Could you check a few things on this model? Use its own coordinates, in mm. A direction names the side the tool comes from. Round coordinates to 2 decimals unless told otherwise and drop trailing zeros. Write each loop counter-clockwise with the first axis right and the second up, starting at its lowest first coordinate (ties: lowest second). Pieces come first, ordered by that corner, then holes. Notation, with made-up numbers: M 5.5,-34 L 41.5,-34 A26 cw 41.5,-12 Z; hole C 82,-19.75 d4. An arc over 180 degrees is marked long. One line per item, written item: value. Start each with the question number.
(1) Thinking about a two-plate mould opening in X: for faces 6 (the face through (-42.005, 1, 0)), 7 (the face through (24.096, 1.493, 21.203)), 8 (the face through (3, 2, -20)), 9 (the face through (41.254, 0.986, 22.962)), which applies, released by +X, released by -X, zero draft, split by the parting line, or undercut?
(2) I'm going to push flat-ended pins straight in: pin 1 Ø0.9 at (x, z) = (-25.5, -20.5) entering from -Y; pin 2 Ø0.8 at (x, y) = (-35.5, 1.5) entering from +Z. Where does each tip first touch, or does it pass through?
(3) I want a section at B-B on z = -6. Please give me the cut outline in (x, y), and give its area (3 significant figures).
(4) If I drill on L1, parallel to X at y = 0.4, z = -9; L2, parallel to Z at x = 12, y = 1.4; L3, parallel to X at y = 1.15, z = 19, over which ranges is the centre line in solid material (lowest first)?
(5) Which directions (+Z, -Z, +X, -X, +Y, -Y) give clear straight access to the entire face, cutting with the end or side of a thin tool? Please do faces 1 (the face through (7, 1, 23.743)), 2 (the face through (-38.63, 1.493, 15.816)), 3 (the face through (1, 1, -22)), 4 (the face through (-41.224, 0.986, 23.002)), 5 (the face through (33.093, 0.986, -17.402)).
(6) I want a section at C-C on y = 0.6. Please give me the cut outline in (x, z).
(7) I want a section at A-A on x = -4.5. Please give me the cut outline in (y, z), and give its area (3 significant figures).
```python
from build123d import *

# Parameters (mm, degrees)
SKETCH_1_R          = 0.9
EXTRUDE_1_DEPTH     = 2
SKETCH_8_W          = 12
SKETCH_8_H          = 10.026739303
CUT_EXTRUDE_4_DEPTH = 1
SKETCH_9_R          = 1.5
CUT_EXTRUDE_7_DEPTH = 1
FILLET_1_R          = 2
SKETCH_10_W         = 12
SKETCH_10_H         = 6.28269209
CUT_EXTRUDE_8_DEPTH = 2
FILLET_2_R          = 1


with BuildPart() as part:
    # 草图1 → 凸台-拉伸1 (new body)
    with BuildSketch(Plane(origin=(0, 0, 0), x_dir=(1, 0, 0), z_dir=(0, 1, 0))):
        with BuildLine():
            Line((-39.407613887, 24.257383456), (39.397836405, 24.257383456))
            ThreePointArc((39.397836405, 24.257383456), (41.234387067, 23.496659264), (41.995111259, 21.660108602))
            Line((41.995111259, 21.660108602), (41.995111259, -21.14534169))
            ThreePointArc((41.995111259, -21.14534169), (41.234387067, -22.981892352), (39.397836405, -23.742616544))
            Line((39.397836405, -23.742616544), (-39.407613887, -23.742616544))
            ThreePointArc((-39.407613887, -23.742616544), (-41.244164549, -22.981892352), (-42.004888741, -21.14534169))
            Line((-42.004888741, -21.14534169), (-42.004888741, 21.660108602))
            ThreePointArc((-42.004888741, 21.660108602), (-41.244164549, 23.496659264), (-39.407613887, 24.257383456))
        make_face()
        with Locations((-25.004888281, 21.257382356)):
            Circle(SKETCH_1_R, mode=Mode.SUBTRACT)
        with Locations((-0.004887481, 21.257382356)):
            Circle(SKETCH_1_R, mode=Mode.SUBTRACT)
        with Locations((24.995110779, 21.257382356)):
            Circle(SKETCH_1_R, mode=Mode.SUBTRACT)
        with Locations((24.995110779, -21.242616464)):
            Circle(SKETCH_1_R, mode=Mode.SUBTRACT)
        with Locations((-0.004887481, -21.242616464)):
            Circle(SKETCH_1_R, mode=Mode.SUBTRACT)
        with Locations((-25.004888281, -21.242616464)):
            Circle(SKETCH_1_R, mode=Mode.SUBTRACT)
        with BuildLine():
            Line((-31.004888741, 18.257383456), (30.995111259, 18.257383456))
            ThreePointArc((30.995111259, 18.257383456), (33.116431602, 17.3787038), (33.995111259, 15.257383456))
            Line((33.995111259, 15.257383456), (33.995111259, -14.742616544))
            ThreePointArc((33.995111259, -14.742616544), (33.116431602, -16.863936887), (30.995111259, -17.742616544))
            Line((30.995111259, -17.742616544), (-31.004888741, -17.742616544))
            ThreePointArc((-31.004888741, -17.742616544), (-33.126209085, -16.863936887), (-34.004888741, -14.742616544))
            Line((-34.004888741, -14.742616544), (-34.004888741, 15.257383456))
            ThreePointArc((-34.004888741, 15.257383456), (-33.126209085, 17.3787038), (-31.004888741, 18.257383456))
        make_face(mode=Mode.SUBTRACT)
    extrude(amount=EXTRUDE_1_DEPTH)

    # 草图8 → 切除-拉伸4 (cut)
    with BuildSketch(Plane(origin=(0, 2, 0), x_dir=(1, 0, 0), z_dir=(0, 1, 0))):
        with Locations((-33.2, -20.228282189)):
            Rectangle(SKETCH_8_W, SKETCH_8_H)
    extrude(amount=-CUT_EXTRUDE_4_DEPTH, mode=Mode.SUBTRACT)

    # 草图9 → 切除-拉伸7 (cut)
    with BuildSketch(Plane.XZ):
        with Locations((-25.004888281, 21.242616464)):
            Circle(SKETCH_9_R)
        with Locations((-0.004887481, 21.242616464)):
            Circle(SKETCH_9_R)
        with Locations((24.995110779, 21.242616464)):
            Circle(SKETCH_9_R)
        with Locations((-25.004888281, -21.257382356)):
            Circle(SKETCH_9_R)
        with Locations((-0.004887481, -21.257382356)):
            Circle(SKETCH_9_R)
        with Locations((24.995110779, -21.257382356)):
            Circle(SKETCH_9_R)
    extrude(amount=-CUT_EXTRUDE_7_DEPTH, mode=Mode.SUBTRACT)

    # 圆角1
    fillet_1_edges = [part.edges().sort_by_distance(p)[0] for p in [
        (-39.2, 1.5, 15.214912538),
    ]]
    fillet(fillet_1_edges, radius=FILLET_1_R)

    # 草图10 → 切除-拉伸8 (cut, through all)
    with BuildSketch(Plane(origin=(0, 1, 0), x_dir=(1, 0, 0), z_dir=(0, 1, 0))):
        with Locations((-33.2, -23.742616544)):
            Rectangle(SKETCH_10_W, SKETCH_10_H)
    extrude(amount=-CUT_EXTRUDE_8_DEPTH, mode=Mode.SUBTRACT)

    # 圆角2
    fillet_2_edges = [part.edges().sort_by_distance(p)[0] for p in [
        (-27.2, 1, 23.742616544),
    ]]
    fillet(fillet_2_edges, radius=FILLET_2_R)


solid = part.part
```
Found:
1. face 6: released by -X
1. face 7: undercut
1. face 8: zero draft
1. face 9: released by +X
2. pin 1: stops at y = 1
2. pin 2: stops at z = 15.21
3. outline: M -42,0 L -34,0 L -34,2 L -42,2 Z; M 34,0 L 42,0 L 42,2 L 34,2 Z
3. area: 32.0 mm²
4. L1: x = -42 to -34, 34 to 42
4. L2: z = -24.26 to -18.26, 17.74 to 23.74
4. L3: x = -42 to -39.2, -27.2 to 42
5. face 1: +Z, +X, -X, +Y, -Y
5. face 2: +Z, +Y
5. face 3: -Y
5. face 4: +Z, -X, +Y, -Y
5. face 5: +Y, -Y
6. outline: M -42,-21.66 A2.6 ccw -39.41,-24.26 L 39.4,-24.26 A2.6 ccw 42,-21.66 L 42,21.15 A2.6 ccw 39.4,23.74 L -26.2,23.74 A1 ccw -27.2,22.74 L -27.2,20.6 L -39.2,20.6 L -39.2,23.74 L -39.41,23.74 A2.6 ccw -42,21.15 Z; hole M -34,-15.26 A3 ccw -31,-18.26 L 31,-18.26 A3 ccw 34,-15.26 L 34,14.74 A3 ccw 31,17.74 L -31,17.74 A3 ccw -34,14.74 Z; hole C -25,-21.26 d3; hole C -25,21.24 d3; hole C 0,-21.26 d3; hole C 0,21.24 d3; hole C 25,-21.26 d3; hole C 25,21.24 d3
7. outline: M 0,-24.26 L 2,-24.26 L 2,-18.26 L 0,-18.26 Z; M 0,17.74 L 2,17.74 L 2,23.74 L 0,23.74 Z
7. area: 24.0 mm²
